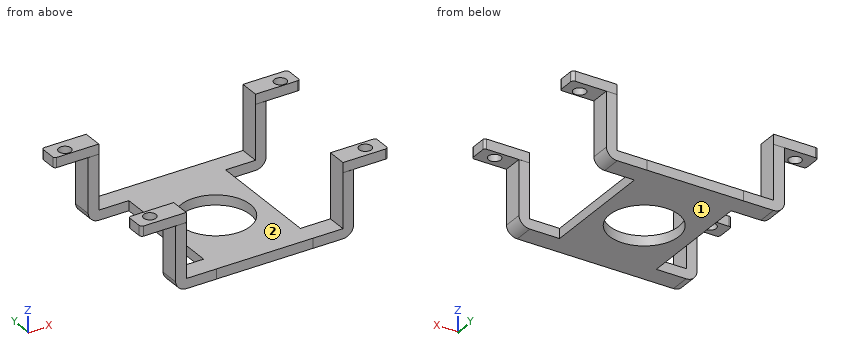
from build123d import *

# Parameters (mm, degrees)
SKETCH076_R  = 7
PAD046_DEPTH = 2
PAD047_DEPTH = 3.99
PAD048_DEPTH = 3.99
SKETCH_R     = 1.25
PAD_DEPTH    = 2


with BuildPart() as pad046:
    # Sketch076 → Pad046 (new body)
    with BuildSketch(Plane.XY.offset(-13)):
        Polygon((-9.775637, 74.2107), (0, 74.2107), (9.775637, 74.2107), (9.775637, 42.511509), (0, 42.511509), (-9.775637, 42.511509), align=None)
        with Locations((0, 58)):
            Circle(SKETCH076_R, mode=Mode.SUBTRACT)
    extrude(amount=-PAD046_DEPTH)


with BuildPart() as pad047:
    # Sketch077 → Pad047 (new body)
    with BuildSketch(Plane.XZ.offset(-42.5)):
        with BuildLine():
            Line((-15.842702, -2), (-18, -2))
            Line((-18, -2), (-18, -13.000001))
            ThreePointArc((-18, -13.000001), (-17.291527, -14.434217), (-15.795265, -15))
            Line((-15.795265, -15), (-9.741142, -15))
            Line((-9.741142, -13), (-9.741142, -15))
            Line((-15.842702, -13), (-9.741142, -13))
            Line((-15.842702, -13), (-15.842702, -2))
        make_face()
        with BuildLine():
            Line((15.842702, -2), (18, -2))
            Line((18, -2), (18, -13.000001))
            ThreePointArc((15.795265, -15), (17.291527, -14.434217), (18, -13.000001))
            Line((15.795265, -15), (9.741142, -15))
            Line((9.741142, -13), (9.741142, -15))
            Line((15.842702, -13), (9.741142, -13))
            Line((15.842702, -13), (15.842702, -2))
        make_face()
    extrude(amount=-PAD047_DEPTH)


with BuildPart() as pad048:
    # Sketch078 → Pad048 (new body)
    with BuildSketch(Plane.XZ.offset(-74.21)):
        with BuildLine():
            Line((-15.842702, -2), (-18, -2))
            Line((-18, -2), (-18, -13.000001))
            ThreePointArc((-18, -13.000001), (-17.291527, -14.434217), (-15.795265, -15))
            Line((-15.795265, -15), (-9.741142, -15))
            Line((-9.741142, -13), (-9.741142, -15))
            Line((-15.842702, -13), (-9.741142, -13))
            Line((-15.842702, -13), (-15.842702, -2))
        make_face()
        with BuildLine():
            Line((15.842702, -2), (18, -2))
            Line((18, -2), (18, -13.000001))
            ThreePointArc((15.795265, -15), (17.291527, -14.434217), (18, -13.000001))
            Line((15.795265, -15), (9.741142, -15))
            Line((9.741142, -13), (9.741142, -15))
            Line((15.842702, -13), (9.741142, -13))
            Line((15.842702, -13), (15.842702, -2))
        make_face()
    extrude(amount=PAD048_DEPTH)


with BuildPart() as battery_holder001:
    # Sketch → Pad (new body)
    with BuildSketch(Plane(origin=(0, 0, 0), x_dir=(-1, 0, 0), z_dir=(0, 0, 1))):
        with BuildLine():
            Line((-25, -43.074277), (-25, -46.007702))
            ThreePointArc((-25, -46.007702), (-24.85848, -46.349363), (-24.516819, -46.490883))
            Line((-15.842702, -46.490883), (-24.516819, -46.490883))
            Line((-15.842702, -42.511509), (-15.842702, -46.490883))
            Line((-24.437232, -42.511509), (-15.842702, -42.511509))
            ThreePointArc((-24.437232, -42.511509), (-24.835169, -42.67634), (-25, -43.074277))
        make_face()
        with Locations((-21.781596, -44.715717)):
            Circle(SKETCH_R, mode=Mode.SUBTRACT)
        with BuildLine():
            Line((-24.842702, -70.71451), (-24.842702, -73.647932))
            ThreePointArc((-24.842702, -73.647932), (-24.677871, -74.045869), (-24.279934, -74.2107))
            Line((-15.842702, -74.2107), (-24.279934, -74.2107))
            Line((-15.842702, -70.23133), (-15.842702, -74.2107))
            Line((-24.359522, -70.23133), (-15.842702, -70.23133))
            ThreePointArc((-24.359522, -70.23133), (-24.701182, -70.37285), (-24.842702, -70.71451))
        make_face()
        with Locations((-21.781596, -71.660071)):
            Circle(SKETCH_R, mode=Mode.SUBTRACT)
        with BuildLine():
            Line((25, -43.074277), (25, -46.007702))
            ThreePointArc((24.516819, -46.490883), (24.85848, -46.349363), (25, -46.007702))
            Line((15.842702, -46.490883), (24.516819, -46.490883))
            Line((15.842702, -42.511509), (15.842702, -46.490883))
            Line((24.437232, -42.511509), (15.842702, -42.511509))
            ThreePointArc((25, -43.074277), (24.835169, -42.67634), (24.437232, -42.511509))
        make_face()
        with Locations((21.781596, -44.715717)):
            Circle(SKETCH_R, mode=Mode.SUBTRACT)
        with BuildLine():
            Line((24.842702, -70.71451), (24.842702, -73.647932))
            ThreePointArc((24.279934, -74.2107), (24.677871, -74.045869), (24.842702, -73.647932))
            Line((15.842702, -74.2107), (24.279934, -74.2107))
            Line((15.842702, -70.23133), (15.842702, -74.2107))
            Line((24.359522, -70.23133), (15.842702, -70.23133))
            ThreePointArc((24.842702, -70.71451), (24.701182, -70.37285), (24.359522, -70.23133))
        make_face()
        with Locations((21.781596, -71.660071)):
            Circle(SKETCH_R, mode=Mode.SUBTRACT)
    extrude(amount=-PAD_DEPTH)

    # Fusion: union Pad046, Pad047, Pad048
    add(pad046.part)
    add(pad047.part)
    add(pad048.part)


solid = battery_holder001.part
Read the model definition and answer for the solid it produces. Units are mm, in the model's axes. Face numbers are marked on the shaded views. Coordinates: 2 decimals unless noted, no trailing zeros. Loops run counter-clockwise (first coordinate to the right, second up) from the corner with the lowest first, then second, coordinate; pieces in that order, holes last. Notation, with made-up numbers: (5, 60.25) - (17, 60.25) arc R21 ccw to (17, 88.25) - close; hole circle Ø3 at (74.25, -14.5). An arc over 180 degrees is marked (long way). Answer in a Markdown table with one row per item.
Q1. Given P1, Ø3, axis at x = -21.78, y = 71.66, coming from the -Z side; P2, Ø2, axis at y = 71.5, z = -1.5, coming from the +X side; P3, Ø10, axis at x = -17.5, y = 55.5, coming from the +Z side; P4, Ø1, axis at y = 60.5, z = -13, coming from the +X side, each flat-ended and moving along its own axis, determine where each tip first touches the part or whether it passes through.
Here are the results:
| item | result |
|---|---|
| P1 | stops at z = -2 |
| P2 | stops at x = 24.84 |
| P3 | passes through |
| P4 | stops at x = 9.78 |
Q2. Find section B-B on x = 0. Write down the section's boundary in (y, z).
Here are the results:
| item | result |
|---|---|
| outline | (42.51, -15) - (51, -15) - (51, -13) - (42.51, -13) - close; (65, -15) - (74.21, -15) - (74.21, -13) - (65, -13) - close |
Q3. Find section A-A on z = -6. Write down the section's boundary in (x, y), plus the area to 3 significant figures.
Here are the results:
| item | result |
|---|---|
| outline | (-18, 42.5) - (-15.84, 42.5) - (-15.84, 46.49) - (-18, 46.49) - close; (-18, 70.22) - (-15.84, 70.22) - (-15.84, 74.21) - (-18, 74.21) - close; (15.84, 42.5) - (18, 42.5) - (18, 46.49) - (15.84, 46.49) - close; (15.84, 70.22) - (18, 70.22) - (18, 74.21) - (15.84, 74.21) - close |
| area | 34.4 mm^2 |
Q4. The mould has two halves that part along X. Classify the marked faces 1 and 2: pulls with the +X half, pulls with the -X half, needs draft (parallel to the pull), parting line crosses it, or undercut.
Here are the results:
| item | result |
|---|---|
| face 1 | needs draft |
| face 2 | undercut |
Q5. Find section C-C on y = 58. Write down the section's boundary in (x, z).
Here are the results:
| item | result |
|---|---|
| outline | (-9.78, -15) - (-7, -15) - (-7, -13) - (-9.78, -13) - close; (7, -15) - (9.78, -15) - (9.78, -13) - (7, -13) - close |
Q6. Find section D-D on x = 22. Write down the section's boundary in (y, z), plus the area to 3 significant figures.
Here are the results:
| item | result |
|---|---|
| outline | (42.51, -2) - (43.48, -2) - (43.48, 0) - (42.51, 0) - close; (45.95, -2) - (46.49, -2) - (46.49, 0) - (45.95, 0) - close; (70.23, -2) - (70.43, -2) - (70.43, 0) - (70.23, 0) - close; (72.89, -2) - (74.21, -2) - (74.21, 0) - (72.89, 0) - close |
| area | 6.07 mm^2 |
Q7. Straight lines are drawn through the part: line 1 along Y through (x, z) = (0, -13.8); line 2 along Y through (x, z) = (21.5, -1.5); line 3 along X through (y, z) = (45.5, -12.5). For each, find the intervals that lie inside material, in ascending order. Write a range as [from, to].
Here are the results:
| item | result |
|---|---|
| line 1 | y = [42.51, 51], [65, 74.21] |
| line 2 | y = [42.51, 43.5], [45.93, 46.49], [70.23, 70.44], [72.88, 74.21] |
| line 3 | x = [-18, -15.84], [15.84, 18] |
